Geometry: see drawing. Coordinates: mm, zero at the bounding-box minimum. A direction names the side the tool comes from. Coordinates: 2 decimals unless noted, no trailing zeros. Order: outer loops, then holes, each group sorted by start corner. A loop starts at its lowest first (then second) coordinate and runs counter-clockwise, first axis right, second up. Notation, with made-up numbers: M 80,36 L 121,36 A6 cw 121,41 Z; hole C 2.5,-36 d5. An arc over 180 degrees is marked long. One line per item, written item: value.
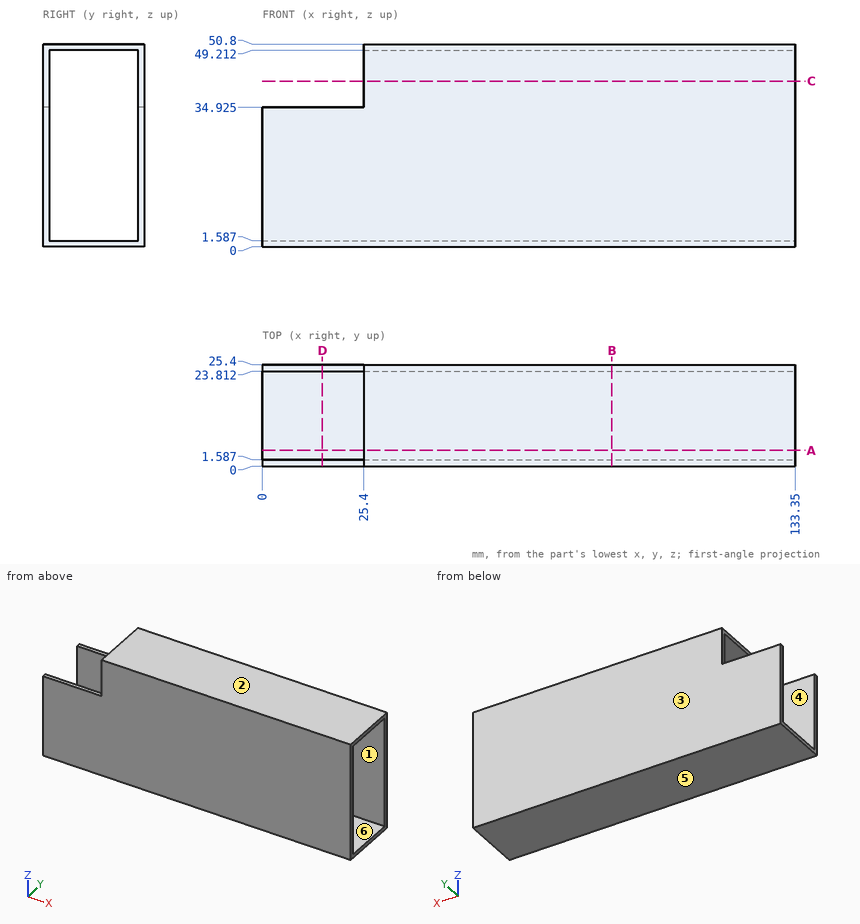
(1) Access query for the marked faces 1 and 2. Directions: +Z, -Z, +X, -X, +Y, -Y. A direction counts if a zero-diameter tool reaches every point of the face in a straight line with its end or side. Return the directions, or none.
Data:
face 1: +X, -X
face 2: +Z, +X, -X, +Y, -Y
(2) Cut plane C-C on z = 41.5. Output: boundary loops of the cut face in (x, y).
Data:
outline: M 25.4,0 L 133.35,0 L 133.35,1.59 L 25.4,1.59 Z; M 25.4,23.81 L 133.35,23.81 L 133.35,25.4 L 25.4,25.4 Z
(3) Cut plane A-A on y = 4. Output: boundary loops of the cut face in (x, z).
Data:
outline: M 0,0 L 133.35,0 L 133.35,1.59 L 0,1.59 Z; M 25.4,49.21 L 133.35,49.21 L 133.35,50.8 L 25.4,50.8 Z
(4) Draft query along Y for the marked faces 3, 4, 5 and 6. Return one class per face: released by +Y, released by -Y, zero draft, split by the parting line, or undercut.
Data:
face 3: released by +Y
face 4: undercut
face 5: zero draft
face 6: undercut
(5) First-contact query: pin 1 (0.8 mm diameter, centred on x = 7.5, y = 24.5, fed in from +Z) (1 decimal). Flat tip, straight axial feed; report the tip coordinate or a pass-through.
Data:
pin 1: stops at z = 34.9
(6) Cut plane D-D on x = 15. Output: boundary loops of the cut face in (y, z) (1 decimal), plus the area to 3 significant figures.
Data:
outline: M 0,0 L 25.4,0 L 25.4,34.9 L 23.8,34.9 L 23.8,1.6 L 1.6,1.6 L 1.6,34.9 L 0,34.9 Z
area: 146 mm2
(7) Ray query, line 1 (Y direction, x = 43.5, z = 49); line 2 (Z direction, x = 28, y = 2); line 3 (Z direction, x = 15.5, y = 19). Return the intervals inside material, ascending. Write a range as from..to.
Data:
line 1: y = 0..1.59, 23.81..25.4
line 2: z = 0..1.59, 49.21..50.8
line 3: z = 0..1.59
(8) Cut plane B-B on x = 87.5. Output: boundary loops of the cut face in (y, z).
Data:
outline: M 0,0 L 25.4,0 L 25.4,50.8 L 0,50.8 Z; hole M 1.59,1.59 L 23.81,1.59 L 23.81,49.21 L 1.59,49.21 Z
